Design review of the part built by this model. Coordinates are the model's own, in mm. A direction names the side the tool comes from. Round coordinates to 2 decimals unless told otherwise and drop trailing zeros. Loops run counter-clockwise (first coordinate to the right, second up) from the corner with the lowest first, then second, coordinate; pieces in that order, holes last. Notation, with made-up numbers: (66.25, 0) -> (97.25, 0) arc R27 cw to (97.25, 18) -> close; hole circle Ø11 at (-16, 0). An arc over 180 degrees is marked (long way). Answer as CSV lines item,"result". Start each with the question number.
```python
from build123d import *

# Parameters (mm, degrees)
SKETCH1_R           = 14.1
SKETCH1_R_2         = 12.6
BOSS_EXTRUDE1_DEPTH = 3.5
SKETCH2_R           = 17.1
SKETCH2_R_2         = 14.1
SKETCH2_R_3         = 12.6
BOSS_EXTRUDE2_DEPTH = 1


with BuildPart() as part:
    # Sketch1 → Boss-Extrude1 (new body)
    with BuildSketch(Plane.XY):
        Circle(SKETCH1_R)
        Circle(SKETCH1_R_2, mode=Mode.SUBTRACT)
    extrude(amount=BOSS_EXTRUDE1_DEPTH)

    # Sketch2 → Boss-Extrude2 (add)
    # profile 1 of 3: a face of its own
    with BuildSketch(Plane.XY.offset(3.5)):
        Circle(SKETCH2_R)
        Circle(SKETCH2_R_2, mode=Mode.SUBTRACT)
    # profile 2 of 3: a face of its own
    with BuildSketch(Plane.XY.offset(3.5)):
        Circle(SKETCH2_R_2)
        Circle(SKETCH2_R_3, mode=Mode.SUBTRACT)
    # profile 3 of 3: a face of its own
    with BuildSketch(Plane.XY.offset(3.5)):
        Circle(SKETCH2_R_3)
    extrude(amount=BOSS_EXTRUDE2_DEPTH)


solid = part.part
```
Q1. Add section C-C, the plane z = 2.55. Give the boundary of the cut face in (x, y), and give its area (3 significant figures).
Q2. For pin 1 Ø1.5 at (x, z) = (-11.5, 4) entering from -Y; pin 2 Ø17 at (x, y) = (0, -3) entering from -Z; pin 3 Ø1 at (x, z) = (-4, 2.5) entering from -Y, all flat-tipped, find the tip position at first contact; note any pin that passes through.
Q3. To check wall thickness, follow probe 1 along Y at (x, z) = (0, 1.05); probe 2 along Z at (x, y) = (-1, 15.5); probe 3 along X at (y, z) = (5, 1). State the ranges of each line that lie inside material, in increasing order. Write a range as from..to.
Q4. Add section A-A, the plane y = 0. Give the boundary of the cut face in (x, z).
Q5. Mouldability with a two-part tool opening along X and no side actions: class faces 1 (the cylindrical face through (-9.999, -7.667, 1.726)), 2 (the flat face through (-11, -7, 0)), 3 (the cylindrical face through (16.31, 5.14, 3.99)), 4 (the flat face through (0, 0, 3.5)) as pulls with the +X half, pulls with the -X half, needs draft (parallel to the pull), parting line crosses it, or undercut.
Q6. Machinability: for faces 5 (the flat face through (-6, 13, 3.5)), 6 (the flat face through (0, 0, 4.5)), which of the approach directions +Z, -Z, +X, -X, +Y, -Y give a long, thin tool a straight path to every point of the face, cutting with its end or side? Answer none if there is none.
Q7. Add section D-D, the plane y = 15.5. Give the boundary of the cut face in (x, z), and give its area (3 significant figures).
Worked answers:
1,outline,"circle Ø28.2 at (0, 0); hole circle Ø25.2 at (0, 0)"
1,area,"126 mm^2"
2,pin 1,"stops at y = -13.3"
2,pin 2,"stops at z = 3.5"
2,pin 3,"stops at y = -13.66"
3,probe 1,"y = -14.1..-12.6, 12.6..14.1"
3,probe 2,"z = 3.5..4.5"
3,probe 3,"x = -13.18..-11.57, 11.57..13.18"
4,outline,"(-17.1, 3.5) -> (-14.1, 3.5) -> (-14.1, 0) -> (-12.6, 0) -> (-12.6, 3.5) -> (12.6, 3.5) -> (12.6, 0) -> (14.1, 0) -> (14.1, 3.5) -> (17.1, 3.5) -> (17.1, 4.5) -> (-17.1, 4.5) -> close"
5,face 1,"undercut"
5,face 2,"needs draft"
5,face 3,"parting line crosses it"
5,face 4,"undercut"
6,face 5,"-Z"
6,face 6,"+Z, +X, -X, +Y, -Y"
7,outline,"(-7.22, 3.5) -> (7.22, 3.5) -> (7.22, 4.5) -> (-7.22, 4.5) -> close"
7,area,"14.4 mm^2"
